Read the model definition and answer for the solid it produces. Units are mm, in the model's axes. A direction names the side the tool comes from. Coordinates: 2 decimals unless noted, no trailing zeros. Loops run counter-clockwise (first coordinate to the right, second up) from the corner with the lowest first, then second, coordinate; pieces in that order, holes last. Notation, with made-up numbers: (3.25, 85) -> (44.25, 85) arc R16 cw to (44.25, 96) -> close; hole circle Ø1 at (79.25, 33). An arc over 180 degrees is marked (long way). One line per question, with ' | ' between items. Start each with the question number.
```python
from build123d import *

# Parameters (mm, degrees)
SKETCH1_W                       = 230
SKETCH1_H                       = 200
EXTRUDE1_DEPTH                  = 5
SKETCH3_R                       = 1.65
SKETCH3_W                       = 60
SKETCH3_H                       = 7
SKETCH3_W_2                     = 13
SKETCH3_H_2                     = 37
EXTRUDE2_DEPTH                  = 5
SKIZZE1_R                       = 1.25
SCHNITT_LINEAR_AUSTRAGEN1_DEPTH = 10
SKIZZE3_R                       = 1.25
SCHNITT_LINEAR_AUSTRAGEN3_DEPTH = 5
SKIZZE4_R                       = 1.65
SKIZZE4_W                       = 5
SKIZZE4_H                       = 10
SCHNITT_LINEAR_AUSTRAGEN4_DEPTH = 10
SKIZZE5_R                       = 1.25
SCHNITT_LINEAR_AUSTRAGEN5_DEPTH = 10
SKIZZE6_W                       = 20.4
SKIZZE6_H                       = 12.9
SCHNITT_LINEAR_AUSTRAGEN6_DEPTH = 10
SKIZZE7_W                       = 10
SKIZZE7_H                       = 10
SCHNITT_LINEAR_AUSTRAGEN7_DEPTH = 10
SKIZZE8_W                       = 10
SKIZZE8_H                       = 10
SCHNITT_LINEAR_AUSTRAGEN8_DEPTH = 10


with BuildPart() as part:
    # Sketch1 → Extrude1 (new body)
    with BuildSketch(Plane(origin=(0, 0, 0), x_dir=(1, 0, 0), z_dir=(0, 1, 0))):
        with Locations((5, 8.694132839)):
            Rectangle(SKETCH1_W, SKETCH1_H)
    extrude(amount=EXTRUDE1_DEPTH)

    # Sketch3 → Extrude2 (cut)
    with BuildSketch(Plane(origin=(0, 5, 0), x_dir=(1, 0, 0), z_dir=(0, 1, 0))):
        with Locations((-86.5, 97.694132839)):
            Circle(SKETCH3_R)
        with Locations((-63.5, 97.694132839)):
            Circle(SKETCH3_R)
        with Locations((-86.5, 69.694132839)):
            Circle(SKETCH3_R)
        with Locations((-63.5, 69.694132839)):
            Circle(SKETCH3_R)
        with Locations((-86.5, -52.305867161)):
            Circle(SKETCH3_R)
        with Locations((-63.5, -52.305867161)):
            Circle(SKETCH3_R)
        with Locations((-86.5, -80.305867161)):
            Circle(SKETCH3_R)
        with Locations((-63.5, -80.305867161)):
            Circle(SKETCH3_R)
        with Locations((73.5, -52.305867161)):
            Circle(SKETCH3_R)
        with Locations((96.5, -52.305867161)):
            Circle(SKETCH3_R)
        with Locations((73.5, -80.305867161)):
            Circle(SKETCH3_R)
        with Locations((96.5, -80.305867161)):
            Circle(SKETCH3_R)
        with Locations((73.5, 97.694132839)):
            Circle(SKETCH3_R)
        with Locations((96.5, 97.694132839)):
            Circle(SKETCH3_R)
        with Locations((73.5, 69.694132839)):
            Circle(SKETCH3_R)
        with Locations((96.5, 69.694132839)):
            Circle(SKETCH3_R)
        with Locations((-36.9, -58.205867161)):
            Circle(SKETCH3_R)
        with Locations((-36.9, 75.594132839)):
            Circle(SKETCH3_R)
        with Locations((47, 75.694132839)):
            Circle(SKETCH3_R)
        with Locations((45, -49.305867161)):
            Circle(SKETCH3_R)
        with Locations((0, 83.694132839)):
            Rectangle(SKETCH3_W, SKETCH3_H)
        with Locations((0, -66.305867161)):
            Rectangle(SKETCH3_W, SKETCH3_H)
        with Locations((-36.5, -28.805867161)):
            Rectangle(SKETCH3_W_2, SKETCH3_H_2)
    extrude(amount=-EXTRUDE2_DEPTH, mode=Mode.SUBTRACT)

    # Skizze1 → Schnitt-Linear austragen1 (cut)
    with BuildSketch(Plane(origin=(0, 5, 0), x_dir=(1, 0, 0), z_dir=(0, 1, 0))):
        with Locations((-102, 100.694132839)):
            Circle(SKIZZE1_R)
        with Locations((-102, -83.305867161)):
            Circle(SKIZZE1_R)
        with Locations((112, -83.305867161)):
            Circle(SKIZZE1_R)
        with Locations((112, 100.694132839)):
            Circle(SKIZZE1_R)
        with Locations((-102, -75.305867161)):
            Circle(SKIZZE1_R)
        with Locations((-102, 92.694132839)):
            Circle(SKIZZE1_R)
        with Locations((112, 92.694132839)):
            Circle(SKIZZE1_R)
        with Locations((112, -75.305867161)):
            Circle(SKIZZE1_R)
    extrude(amount=-SCHNITT_LINEAR_AUSTRAGEN1_DEPTH, mode=Mode.SUBTRACT)

    # Skizze3 → Schnitt-Linear austragen3 (cut)
    with BuildSketch(Plane(origin=(0, 5, 0), x_dir=(1, 0, 0), z_dir=(0, 1, 0))):
        with Locations((-8.221682518, -77.643318078)):
            Circle(SKIZZE3_R)
        with Locations((47.278317482, -77.643318078)):
            Circle(SKIZZE3_R)
    extrude(amount=-SCHNITT_LINEAR_AUSTRAGEN3_DEPTH, mode=Mode.SUBTRACT)

    # Skizze4 → Schnitt-Linear austragen4 (cut)
    with BuildSketch(Plane(origin=(0, 5, 0), x_dir=(1, 0, 0), z_dir=(0, 1, 0))):
        with Locations((112.5, 23.694132839)):
            Circle(SKIZZE4_R)
        with Locations((112.5, -6.305867161)):
            Circle(SKIZZE4_R)
        with Locations((-102.5, 23.694132839)):
            Circle(SKIZZE4_R)
        with Locations((-102.5, -6.305867161)):
            Circle(SKIZZE4_R)
        with Locations((110.5, -23.305867161)):
            Rectangle(SKIZZE4_W, SKIZZE4_H)
        with Locations((110.5, 40.694132839)):
            Rectangle(SKIZZE4_W, SKIZZE4_H)
        with Locations((-100.5, 40.694132839)):
            Rectangle(SKIZZE4_W, SKIZZE4_H)
        with Locations((-100.5, -23.305867161)):
            Rectangle(SKIZZE4_W, SKIZZE4_H)
    extrude(amount=-SCHNITT_LINEAR_AUSTRAGEN4_DEPTH, mode=Mode.SUBTRACT)

    # Skizze5 → Schnitt-Linear austragen5 (cut)
    with BuildSketch(Plane(origin=(0, 5, 0), x_dir=(1, 0, 0), z_dir=(0, 1, 0))):
        with Locations((100, 18.694132839)):
            Circle(SKIZZE5_R)
        with Locations((100, -1.305867161)):
            Circle(SKIZZE5_R)
        with Locations((30, 18.694132839)):
            Circle(SKIZZE5_R)
        with Locations((30, -1.305867161)):
            Circle(SKIZZE5_R)
    extrude(amount=-SCHNITT_LINEAR_AUSTRAGEN5_DEPTH, mode=Mode.SUBTRACT)

    # Skizze6 → Schnitt-Linear austragen6 (cut)
    with BuildSketch(Plane(origin=(0, 5, 0), x_dir=(1, 0, 0), z_dir=(0, 1, 0))):
        with Locations((29.8, -29.855867161)):
            Rectangle(SKIZZE6_W, SKIZZE6_H)
    extrude(amount=-SCHNITT_LINEAR_AUSTRAGEN6_DEPTH, mode=Mode.SUBTRACT)

    # Skizze7 → Schnitt-Linear austragen7 (cut)
    with BuildSketch(Plane(origin=(0, 5, 0), x_dir=(1, 0, 0), z_dir=(0, 1, 0))):
        with Locations((-75, 8.694132839)):
            Rectangle(SKIZZE7_W, SKIZZE7_H)
    extrude(amount=-SCHNITT_LINEAR_AUSTRAGEN7_DEPTH, mode=Mode.SUBTRACT)

    # Skizze8 → Schnitt-Linear austragen8 (cut)
    with BuildSketch(Plane(origin=(0, 5, 0), x_dir=(1, 0, 0), z_dir=(0, 1, 0))):
        with Locations((50, 50.694132839)):
            Rectangle(SKIZZE8_W, SKIZZE8_H)
        with Locations((50, -28.305867161)):
            Rectangle(SKIZZE8_W, SKIZZE8_H)
    extrude(amount=-SCHNITT_LINEAR_AUSTRAGEN8_DEPTH, mode=Mode.SUBTRACT)


solid = part.part
```
(1) A tool of negligible diameter and unlimited length cuts with its end or side. For faces 3 (the flat face through (55, 3, -51)), 4 (the flat face through (3, 0, -10)), from which of +Z, -Z, +X, -X, +Y, -Y can it reach the whole face along a straight path? Write none if from no direction.
(2) Determine the mould class of faces 1 (the flat face through (-80, 3, -9)), 2 (the flat face through (120, 2, -7)) for opening direction Z: +Z half, -Z half, draft (parallel to the pull), parting line (faces both ways), or undercut.
(3) Section B-B on x = -25.5 is taken. Write down the section's boundary in (y, z).
(4) Find the intervals of material crossed by probe 1 along Z at (x, y) = (-22, 4.55); probe 2 along Z at (x, y) = (52, 0.9); probe 3 along Z at (x, y) = (-63.5, 3.3), in increasing order. Write a range as from..to.
(5) Section C-C on y = 2.8 is taken. Give the number of separate pieces and of enclosed holes in the cut face, plus the area to 3 significant figures.
(6) This flat-tipped pin is pushed along its axis until it touches: pin 1 Ø1 at (x, z) = (49, -16.5) entering from -Y. Where does it stop, or does it pass through?
(7) Section A-A on z = -39 is taken. Write down the section's boundary in (x, y).
Working result:
1) face 3: +Y, -Y | face 4: +Z, -Z, +X, -X, -Y
2) face 1: undercut | face 2: draft
3) outline: (0, -108.69) -> (5, -108.69) -> (5, -87.19) -> (0, -87.19) -> close; (0, -80.19) -> (5, -80.19) -> (5, 62.81) -> (0, 62.81) -> close; (0, 69.81) -> (5, 69.81) -> (5, 91.31) -> (0, 91.31) -> close
4) probe 1: z = -108.69..-87.19, -80.19..62.81, 69.81..91.31 | probe 2: z = -108.69..-55.69, -45.69..23.31, 33.31..91.31 | probe 3: z = -108.69..-99.34, -96.04..-71.34, -68.04..50.66, 53.96..78.66, 81.96..91.31
5) separate pieces: 1 | enclosed holes: 49 | area: 43,600 mm2
6) pin 1: stops at y = 0
7) outline: (-110, 0) -> (-103, 0) -> (-103, 5) -> (-110, 5) -> close; (-98, 0) -> (108, 0) -> (108, 5) -> (-98, 5) -> close; (113, 0) -> (120, 0) -> (120, 5) -> (113, 5) -> close
